Input: part model. Units: mm. Frame: model coordinates. A direction names the side the tool comes from. Round coordinates to 2 decimals unless told otherwise and drop trailing zeros. Loops run counter-clockwise (first coordinate to the right, second up) from the corner with the lowest first, then second, coordinate; pieces in that order, holes last. Notation, with made-up numbers: M 72.5,-18.5 L 117.5,-18.5 A13 ccw 117.5,-7.5 Z; hole C -16.75,28 d2. An arc over 180 degrees is marked long. Put each result on its own line as item: value. Start each with the question number.
1) Reachability of faces 4 (the face through (-1.888, 14.377, 4.93)), 5 (the face through (-14.5, -22, 9)) from +Z, -Z, +X, -X, +Y, -Y: full face, straight path, thin tool, end or side. Return the list, or none.
2) Line query: probe 1 along Y at (x, z) = (0, 6.5); probe 2 along X at (y, z) = (-0.5, 2.25); probe 3 along Y at (x, z) = (0, 1.45). Output: solid intervals per line, ascending.
3) Section C-C on y = 2. Output: boundary loops of the cut face in (x, z), plus the area to 3 significant figures.
4) Draft query along Y for faces 1 (the face through (0.203, -25.787, 0.601)), 2 (the face through (0, -21.457, 13)), 3 (the face through (6, -12, 10)). Return one class per face: +Y half, -Y half, draft (parallel to the pull), parting line (faces both ways), or undercut.
5) Section D-D on x = 7.5. Output: boundary loops of the cut face in (y, z), plus the area to 3 significant figures.
6) Section B-B on x = 0. Output: boundary loops of the cut face in (y, z), plus the area to 3 significant figures.
7) Pin query (flat end, axial travel): pin 1 (17 mm diameter, centred on x = 6, y = -7, fed in from +Z); pin 2 (1 mm diameter, centred on x = -7.5, z = 4, fed in from +Y); pin 3 (10 mm diameter, centred on x = 6.5, y = -20, fed in from +Z); pin 4 (10 mm diameter, centred on x = 9.5, z = 10, fed in from +Y). Return the tip coordinate at first contact, or that it passes through.
8) Section A-A on z = 8. Output: boundary loops of the cut face in (x, y).
from build123d import *

# Parameters (mm, degrees)
F0_R     = 13.25
F1_DEPTH = 10
F0_R_2   = 1
F0_W     = 29
F0_H     = 4.9
F2_DEPTH = 2
F3_DEPTH = 25
F4_R     = 2


with BuildPart() as f1:
    # F0 (on Top) → F1 (new body)
    with BuildSketch(Plane.XY):
        with BuildLine():
            ThreePointArc((-14.5, 0), (0, -14.5), (14.5, 0))
            ThreePointArc((14.5, 0), (0, 14.5), (-14.5, 0))
        make_face()
        Circle(F0_R, mode=Mode.SUBTRACT)
    extrude(amount=F1_DEPTH)

    # F0 (on Top) → F2 (join)
    with BuildSketch(Plane.XY):
        with BuildLine():
            Line((14.5, -21.457395), (14.5, 0))
            ThreePointArc((14.5, 0), (0, -14.5), (-14.5, 0))
            Line((-14.5, 0), (-14.5, -21.457395))
            Line((-14.5, -21.457395), (14.5, -21.457395))
        make_face()
        with Locations((0, -18.957395)):
            Circle(F0_R_2, mode=Mode.SUBTRACT)
        with Locations((0, -23.907395)):
            Rectangle(F0_W, F0_H)
    extrude(amount=F2_DEPTH)

    # F0 (on Top) → F3 (join)
    with BuildSketch(Plane.XY):
        with Locations((0, -23.907395)):
            Rectangle(F0_W, F0_H)
    extrude(amount=F3_DEPTH)

    # F4
    f4_edges = [f1.edges().sort_by_distance(p)[0] for p in [
        (0, -26.357395, 0),
    ]]
    fillet(f4_edges, radius=F4_R)


solid = f1.part
Geometry results:
1. face 4: +Z
1. face 5: +Z, -Z, -X, +Y, -Y
2. probe 1: y = -26.36 to -21.46, -14.5 to -13.25, 13.25 to 14.5
2. probe 2: x = -14.49 to -13.24, 13.24 to 14.49
2. probe 3: y = -26.28 to -19.96, -17.96 to -13.25, 13.25 to 14.5
3. outline: M -14.36,0 L -13.1,0 L -13.1,10 L -14.36,10 Z; M 13.1,0 L 14.36,0 L 14.36,10 L 13.1,10 Z
3. area: 25.3 mm²
4. face 1: -Y half
4. face 2: undercut
4. face 3: draft
5. outline: M -26.36,2 A2 ccw -24.36,0 L -10.92,0 L -10.92,10 L -12.41,10 L -12.41,2 L -21.46,2 L -21.46,25 L -26.36,25 Z; M 10.92,0 L 12.41,0 L 12.41,10 L 10.92,10 Z
5. area: 169 mm²
6. outline: M -26.36,2 A2 ccw -24.36,0 L -19.96,0 L -19.96,2 L -21.46,2 L -21.46,25 L -26.36,25 Z; M -17.96,0 L -13.25,0 L -13.25,10 L -14.5,10 L -14.5,2 L -17.96,2 Z; M 13.25,0 L 14.5,0 L 14.5,10 L 13.25,10 Z
6. area: 157 mm²
7. pin 1: stops at z = 10
7. pin 2: stops at y = 12.7
7. pin 3: stops at z = 25
7. pin 4: stops at y = 13.78
8. outline: M -14.5,-26.36 L 14.5,-26.36 L 14.5,-21.46 L -14.5,-21.46 Z; C 0,0 d29; hole C 0,0 d26.5
